Print and shaded views of the part. All mm, measured from the part's lowest x, y and z. A direction names the side the tool comes from. Give positions to 0.01 mm unless a question says otherwise; leave off trailing zeros. Order: outer loops, then holes, each group sorted by start corner. A loop starts at its lowest first (then second) coordinate and runs counter-clockwise, first axis right, second up. Notation, with made-up numbers: (31, 10) - (60, 10) arc R13 ccw to (60, 19) - close; hole circle Ø4 at (-22, 70.5). An arc over 180 degrees is marked (long way). Answer in a Markdown table with one row per item.
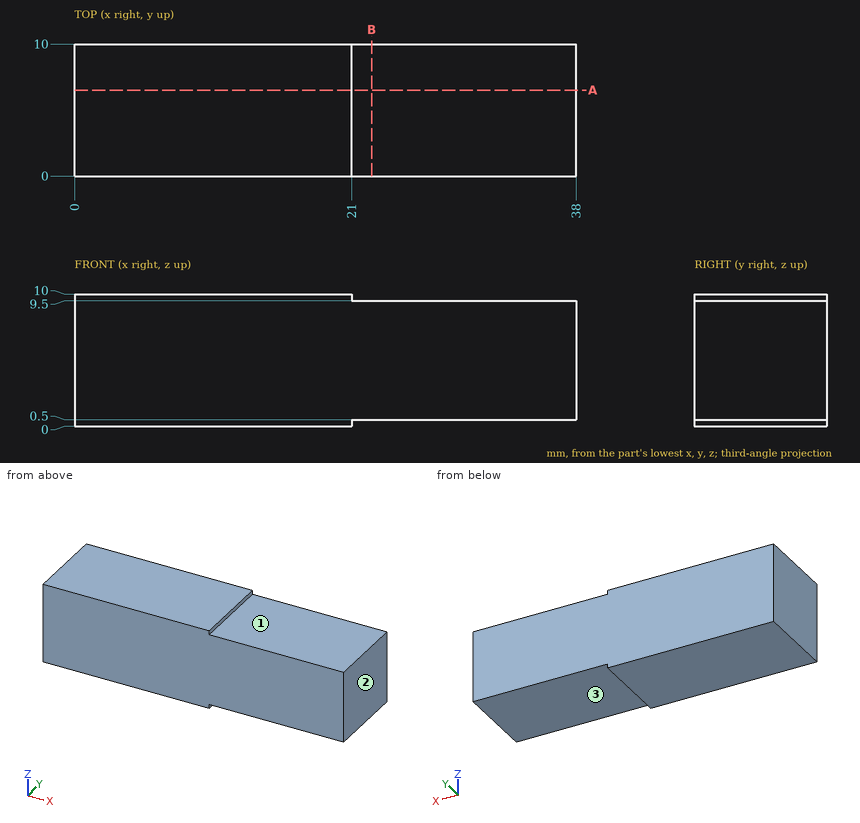
1. Probe line 1 (Z direction, x = 26, y = 4.5); line 2 (X direction, y = 4.75, z = 9.75). List the from-to ranges inside material, lowest first.
Check result:
| item | result |
|---|---|
| line 1 | z = 0.5 to 9.5 |
| line 2 | x = 0 to 21 |
2. Cut at B-B on x = 22.5. Write the cut outline in (y, z), and give its area (3 significant figures).
Check result:
| item | result |
|---|---|
| outline | (0, 0.5) - (10, 0.5) - (10, 9.5) - (0, 9.5) - close |
| area | 90.0 mm² |
3. Drop flat-ended pins along their axis: P1, Ø1, axis at y = 1.5, z = 6, coming from the -X side; P2, Ø5, axis at x = 28.5, y = 3, coming from the -Z side. Give the stop position or say it passes through.
Check result:
| item | result |
|---|---|
| P1 | stops at x = 0 |
| P2 | stops at z = 0.5 |
4. Cut at A-A on y = 6.5. Write the cut outline in (x, z).
Check result:
| item | result |
|---|---|
| outline | (0, 0) - (21, 0) - (21, 0.5) - (38, 0.5) - (38, 9.5) - (21, 9.5) - (21, 10) - (0, 10) - close |
5. Which spindle directions (+Z, -Z, +X, -X, +Y, -Y) get a long thin tool onto all of the face, cutting with end or side? Do the marked faces 1, 2 and 3. Say none if no direction does.
Check result:
| item | result |
|---|---|
| face 1 | +Z, +X, +Y, -Y |
| face 2 | +Z, -Z, +X, +Y, -Y |
| face 3 | -Z, +X, +Y, -Y |
